Source: CAD feature listing. Evaluate the final solid. Frame: model axes, mm. Face numbers are marked on the shaded views. A direction names the side the tool comes from. Round coordinates to 2 decimals unless told otherwise and drop trailing zeros. Order: outer loops, then holes, each group sorted by start corner. A loop starts at its lowest first (then second) coordinate and runs counter-clockwise, first axis right, second up. Notation, with made-up numbers: (89, 84.25) - (140, 84.25) arc R7 cw to (140, 88.25) - close; hole circle Ø3 at (54.25, -15.75). An arc over 180 degrees is marked (long way). Return JSON: item names as keys, results as strings. Group by question number.
1) Mould query, pull axis X, two halves, no side actions, for the marked faces 5, 6, 7 and 8. Classes: pulls with the +X half, pulls with the -X half, needs draft (parallel to the pull), parting line crosses it, or undercut.
2) Section A-A, the plane x = 0. Return loops of the section in (y, z).
3) Ray query, line 1 (Y direction, x = 5, z = -1.75); line 2 (Y direction, x = 2.75, z = -3.5); line 3 (X direction, y = 3.5, z = 0). Return the intervals inside material, ascending. Write a range as from..to.
4) Section D-D, the plane y = 22. Return loops of the section in (x, z).
5) Section C-C, the plane y = 10.5. Return loops of the section in (x, z), plus the area to 3 significant figures.
6) Contact query for flat-ended pins moving along their axis: P1, Ø0.6, axis at y = -4, z = 0, coming from the -X side; P2, Ø3, axis at x = -1.5, y = 18, coming from the +Z side; P3, Ø2, axis at y = -1.5, z = 0.5, coming from the +X side. Output: stop coordinate, or through.
7) Access query for the marked faces 1, 2, 3 and 4. Directions: +Z, -Z, +X, -X, +Y, -Y. A direction counts if a zero-diameter tool reaches every point of the face in a straight line with its end or side. Return the directions, or none.
```python
from build123d import *

# Parameters (mm, degrees)
BOSS_EXTRU_1_DEPTH      = 1
BOSS_EXTRU_1_DEPTH_BACK = 1
ESQUISSE2_W             = 0.5
ESQUISSE2_H             = 5.8
CONG_2_R                = 0.4


with BuildPart() as part:
    # Esquisse1 → R_volution1 (revolve)
    with BuildSketch(Plane.XY, mode=Mode.PRIVATE) as r_volution1_sk:
        Polygon((0, 0), (0, 24.3), (-1.8, 24.3), (-1.8, 20), (-2.4, 20), (-2.4, 15.7), (-3.5, 15.7), (-3.5, 9.7), (-5.5, 9.7), (-5.5, 8.9), (-5, 8.9), (-5, 6), (-4, 6), (-4, 0), align=None)
    revolve(r_volution1_sk.sketch.rotate(Axis((0, 0, 0), (0, 1, 0)), 270), axis=Axis((0, 0, 0), (0, 1, 0)))

    # Esquisse2 → Boss.-Extru.1 (add, two sides: drawn at the far end of the back side and taken through both)
    with BuildSketch(Plane.XY.offset(-BOSS_EXTRU_1_DEPTH_BACK)):
        with Locations((-2, -2.9)):
            Rectangle(ESQUISSE2_W, ESQUISSE2_H)
        with Locations((2, -2.9)):
            Rectangle(ESQUISSE2_W, ESQUISSE2_H)
    extrude(amount=BOSS_EXTRU_1_DEPTH + BOSS_EXTRU_1_DEPTH_BACK)

    # Cong_2
    cong_2_edges = [part.edges().sort_by_distance(p)[0] for p in [
        (-2, -5.8, -1),
        (-2, -5.8, 1),
        (2, -5.8, -1),
        (2, -5.8, 1),
    ]]
    fillet(cong_2_edges, radius=CONG_2_R)


solid = part.part
```
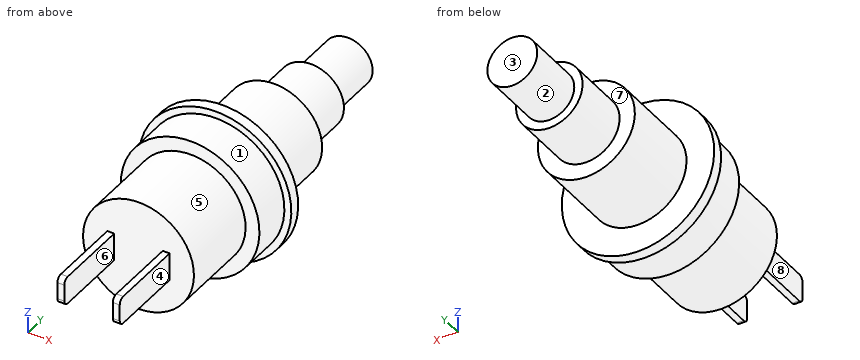
Geometry check:
{
 "1": {"face 5": "parting line crosses it", "face 6": "undercut", "face 7": "needs draft", "face 8": "pulls with the -X half"},
 "2": {"outline": "(0, -4) - (6, -4) - (6, -5) - (8.9, -5) - (8.9, -5.5) - (9.7, -5.5) - (9.7, -3.5) - (15.7, -3.5) - (15.7, -2.4) - (20, -2.4) - (20, -1.8) - (24.3, -1.8) - (24.3, 1.8) - (20, 1.8) - (20, 2.4) - (15.7, 2.4) - (15.7, 3.5) - (9.7, 3.5) - (9.7, 5.5) - (8.9, 5.5) - (8.9, 5) - (6, 5) - (6, 4) - (0, 4) - close"},
 "3": {"line 1": "8.9..9.7", "line 2": "6..9.7", "line 3": "-4..4"},
 "4": {"outline": "circle Ø3.6 at (0, 0)"},
 "5": {"outline": "circle Ø7 at (0, 0)", "area": "38.5 mm2"},
 "6": {"P1": "x = -2.25", "P2": "z = 2.4", "P3": "x = 2.25"},
 "7": {"face 1": "-Y", "face 2": "+Y", "face 3": "+Z, -Z, +X, -X, +Y", "face 4": "+Z, -Z, +X, -Y"}
}
